For this review, take the finished solid that the model builds, in its own axes (mm). Face numbers are marked on the shaded views. A direction names the side the tool comes from. Coordinates: 2 decimals unless noted, no trailing zeros. Write each loop counter-clockwise with the first axis right and the second up, starting at its lowest first coordinate (ties: lowest second). Pieces come first, ordered by that corner, then holes. Notation, with made-up numbers: (18.5, -27.75) - (47.5, -27.75) arc R26 cw to (47.5, 3.25) - close; hole circle Ø6 at (35.5, 51). An arc over 180 degrees is marked (long way). Use one line per item in the form item = value. Start each with the question number.
1) For L1, parallel to X at y = 4, z = 0.5; L2, parallel to Y at x = 1.6, z = 0.55; L3, parallel to Z at x = -2, y = 26, list the stretches that pass through material, from the lowest coordinate up. Write a range as from..to.
2) We need section B-B (x = 0). Give the boundary of the cut face in (y, z), plus the area to 3 significant figures.
3) Insertion check: P1, Ø2.5, axis at y = 0, z = -0.5, coming from the +X side; P2, Ø0.8, axis at y = -6.5, z = 0, coming from the +X side; P3, Ø1, axis at x = -1.5, y = 24, coming from the -Z side. Each pin has a flat end and moves straight along its axis. Give the tip position at first contact, or say it passes through.
4) We need section D-D (y = -1). Give the boundary of the cut face in (x, z).
5) We need section A-A (z = 0). Give the boundary of the cut face in (x, y), plus the area to 3 significant figures.
6) Tool access review of the marked faces 1, 2 and 3: name each direction out of +Z, -Z, +X, -X, +Y, -Y from which nothing blocks a thin tool from reaching the whole face with its end or side.
7) We need section C-C (y = 16.5). Give the boundary of the cut face in (x, z).
```python
from build123d import *

# Parameters (mm, degrees)
SKETCH1_R           = 2.5
BOSS_EXTRUDE1_DEPTH = 50
BOSS_EXTRUDE2_START = 8.295452371
SKETCH2_R           = 2.5
BOSS_EXTRUDE2_DEPTH = 8.295452371
SKETCH4_OUTSIDE_W   = 18.744
SKETCH4_OUTSIDE_H   = 18.744
CUT_EXTRUDE1_DEPTH  = 3.6
CUT_EXTRUDE2_DEPTH  = 10
CUT_EXTRUDE3_START  = -20
SKETCH7_R           = 2.5
CUT_EXTRUDE3_DEPTH  = 20


with BuildPart() as part:
    # Sketch1 → Boss-Extrude1 (new body)
    with BuildSketch(Plane(origin=(0, 0, 0), x_dir=(1, 0, 0), z_dir=(0, 1, 0))):
        with Locations(Location((0, 0, 0), (0, 0, 270))):
            Circle(SKETCH1_R)
    extrude(amount=BOSS_EXTRUDE1_DEPTH)

    # Sketch2 → Boss-Extrude2 (add)
    with BuildSketch(Plane(origin=(0, 0, 0), x_dir=(-1, 0, 0), z_dir=(0, -1, 0)).offset(BOSS_EXTRUDE2_START)):
        with Locations(Location((0, 0, 0), (0, 0, 270))):
            Circle(SKETCH2_R)
    extrude(amount=-BOSS_EXTRUDE2_DEPTH)

    # Sketch4 outside → Cut-Extrude1 (cut)
    with BuildSketch(Plane.XZ.offset(8.295452371)):
        Rectangle(SKETCH4_OUTSIDE_W, SKETCH4_OUTSIDE_H)
        with BuildLine():
            Line((1.25, 0.75), (1.25, -0.75))
            ThreePointArc((1.25, -0.75), (0, -2), (-1.25, -0.75))
            Line((-1.25, -0.75), (-1.25, 0.75))
            ThreePointArc((-1.25, 0.75), (0, 2), (1.25, 0.75))
        make_face(mode=Mode.SUBTRACT)
    extrude(amount=-CUT_EXTRUDE1_DEPTH, mode=Mode.SUBTRACT)

    # Sketch5 → Cut-Extrude2 (cut)
    with BuildSketch(Plane(origin=(0, -4.695452371, 0), x_dir=(-1, 0, 0), z_dir=(0, -1, 0))):
        with BuildLine():
            Line((2, -1.5), (2, 1.5))
            ThreePointArc((2, 1.5), (2.5, 0), (2, -1.5))
        make_face()
        with BuildLine():
            Line((-2, -1.5), (-2, 1.5))
            ThreePointArc((-2, 1.5), (-2.5, 0), (-2, -1.5))
        make_face()
    extrude(amount=-CUT_EXTRUDE2_DEPTH, mode=Mode.SUBTRACT)

    # Sketch7 → Cut-Extrude3 (cut)
    with BuildSketch(Plane(origin=(0, 50, 0), x_dir=(1, 0, 0), z_dir=(0, 1, 0)).offset(CUT_EXTRUDE3_START)):
        with Locations(Location((0, 0, 0), (0, 0, 143.130102354))):
            Circle(SKETCH7_R)
    extrude(amount=CUT_EXTRUDE3_DEPTH, mode=Mode.SUBTRACT)


solid = part.part
```
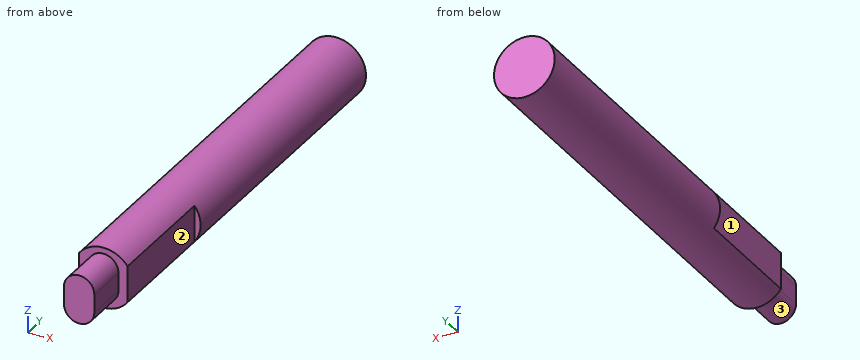
Determined:
q1.L1 = -2..2
q1.L2 = -4.7..30
q1.L3 = -1.5..1.5
q2.outline = (-8.3, -2) - (-4.7, -2) - (-4.7, -2.5) - (30, -2.5) - (30, 2.5) - (-4.7, 2.5) - (-4.7, 2) - (-8.3, 2) - close
q2.area = 188 mm²
q3.P1 = 2
q3.P2 = 1.25
q3.P3 = -2.29
q4.outline = (-2, -1.5) arc R2.5 ccw to (2, -1.5) - (2, 1.5) arc R2.5 ccw to (-2, 1.5) - close
q5.outline = (-2.5, 5.3) - (-2, 5.3) - (-2, -4.7) - (-1.25, -4.7) - (-1.25, -8.3) - (1.25, -8.3) - (1.25, -4.7) - (2, -4.7) - (2, 5.3) - (2.5, 5.3) - (2.5, 30) - (-2.5, 30) - close
q5.area = 172 mm²
q6.face_1 = +Z, -Z, -X, -Y
q6.face_2 = +Z, -Z, +X, -Y
q6.face_3 = -Z, -Y
q7.outline = circle Ø5 at (0, 0)
